The model under review builds one solid part; all positions refer to its coordinate system, in mm. A direction names the side the tool comes from. Give positions to 0.01 mm unless a question says otherwise; leave off trailing zeros. Loops run counter-clockwise (first coordinate to the right, second up) from the corner with the lowest first, then second, coordinate; pieces in that order, holes last. Notation, with made-up numbers: M 32,3 L 47,3 A31 cw 47,38 Z; hole C -5.75,78.25 d2. An arc over 180 degrees is marked long. Return JSON: item names as keys, results as strings. Group by question number.
```python
from build123d import *

# Parameters (mm, degrees)
CUT_EXTRUDE1_START     = -5
CUT_EXTRUDE1_OUTLINE_R = 1.75
CUT_EXTRUDE1_OUTLINE_W = 20.75
CUT_EXTRUDE1_OUTLINE_H = 41.25
CUT_EXTRUDE1_DEPTH     = 5
BOSS_EXTRUDE1_START    = -5
BOSS_EXTRUDE1_DEPTH    = 5
SKETCH4_W              = 30
SKETCH4_H              = 60
BOSS_EXTRUDE2_DEPTH    = 5
CUT_EXTRUDE2_REACH     = 160.193
SKETCH5_W              = 4.2
SKETCH5_H              = 20
CUT_EXTRUDE3_REACH     = 160.193
SKETCH6_R              = 1.75


with BuildPart() as part:
    # Cut-Extrude1: read off the stored shape, not the designer's step
    # Cut-Extrude1 outline → Cut-Extrude1 (new body)
    with BuildSketch(Plane(origin=(5, 0, 0), x_dir=(0, 0, -1), z_dir=(1, 0, 0)).offset(CUT_EXTRUDE1_START)):
        with BuildLine():
            Line((-6.17, -30), (6.17, -30))
            ThreePointArc((6.17, -30), (12.413752878, -27.413752878), (15, -21.17))
            Line((15, -21.17), (15, 21.17))
            ThreePointArc((15, 21.17), (12.413752878, 27.413752878), (6.17, 30))
            Line((6.17, 30), (-6.17, 30))
            ThreePointArc((-6.17, 30), (-12.413752878, 27.413752878), (-15, 21.17))
            Line((-15, 21.17), (-15, -21.17))
            ThreePointArc((-15, -21.17), (-12.413752878, -27.413752878), (-6.17, -30))
        make_face()
        with Locations((-4.875, -24.3)):
            Circle(CUT_EXTRUDE1_OUTLINE_R, mode=Mode.SUBTRACT)
        with Locations((4.875, -24.3)):
            Circle(CUT_EXTRUDE1_OUTLINE_R, mode=Mode.SUBTRACT)
        with Locations((-4.875, 24.3)):
            Circle(CUT_EXTRUDE1_OUTLINE_R, mode=Mode.SUBTRACT)
        Rectangle(CUT_EXTRUDE1_OUTLINE_W, CUT_EXTRUDE1_OUTLINE_H, mode=Mode.SUBTRACT)
        with Locations((4.875, 24.3)):
            Circle(CUT_EXTRUDE1_OUTLINE_R, mode=Mode.SUBTRACT)
    extrude(amount=CUT_EXTRUDE1_DEPTH)

    # Sketch2 → Boss-Extrude1 (add)
    with BuildSketch(Plane(origin=(5, 0, 0), x_dir=(0, 0, -1), z_dir=(1, 0, 0)).offset(BOSS_EXTRUDE1_START)):
        with BuildLine():
            Line((10.375, -20.625), (6.17, -20.625))
            Line((6.17, -20.625), (6.17, -21.93080825))
            Line((6.17, -21.93080825), (7.268440243, -21.93080825))
            Line((7.268440243, -21.93080825), (7.268440243, -27.341819789))
            Line((7.268440243, -27.341819789), (6.17, -27.341819789))
            Line((6.17, -27.341819789), (6.17, -30))
            ThreePointArc((6.17, -30), (12.413752878, -27.413752878), (15, -21.17))
            Line((15, -21.17), (15, 21.17))
            ThreePointArc((15, 21.17), (12.413752878, 27.413752878), (6.17, 30))
            Line((6.17, 30), (6.17, 26.982507006))
            Line((6.17, 26.982507006), (7.710578553, 26.982507006))
            Line((7.710578553, 26.982507006), (7.710578553, 21.584637872))
            Line((7.710578553, 21.584637872), (6.17, 21.584637872))
            Line((6.17, 21.584637872), (6.17, 20.625))
            Line((6.17, 20.625), (10.375, 20.625))
            Line((10.375, 20.625), (10.375, -20.625))
        make_face()
        with BuildLine():
            Line((-8.472684232, -21.93080825), (-6.17, -21.93080825))
            Line((-6.17, -21.93080825), (-6.17, -20.625))
            Line((-6.17, -20.625), (-10.375, -20.625))
            Line((-10.375, -20.625), (-10.375, 20.625))
            Line((-10.375, 20.625), (-6.17, 20.625))
            Line((-6.17, 20.625), (-6.17, 21.584637872))
            Line((-6.17, 21.584637872), (-7.710578553, 21.584637872))
            Line((-7.710578553, 21.584637872), (-7.710578553, 26.982507006))
            Line((-7.710578553, 26.982507006), (-6.17, 26.982507006))
            Line((-6.17, 26.982507006), (-6.17, 30))
            ThreePointArc((-6.17, 30), (-12.413752878, 27.413752878), (-15, 21.17))
            Line((-15, 21.17), (-15, -21.17))
            ThreePointArc((-15, -21.17), (-12.413752878, -27.413752878), (-6.17, -30))
            Line((-6.17, -30), (-6.17, -27.341819789))
            Line((-6.17, -27.341819789), (-8.472684232, -27.341819789))
            Line((-8.472684232, -27.341819789), (-8.472684232, -21.93080825))
        make_face()
        with BuildLine():
            Line((-15, 30), (-15, 21.17))
            ThreePointArc((-15, 21.17), (-12.413752878, 27.413752878), (-6.17, 30))
            Line((-6.17, 30), (-15, 30))
        make_face()
        with BuildLine():
            Line((15, 30), (6.17, 30))
            ThreePointArc((6.17, 30), (12.413752878, 27.413752878), (15, 21.17))
            Line((15, 21.17), (15, 30))
        make_face()
        with BuildLine():
            ThreePointArc((15, -21.17), (12.413752878, -27.413752878), (6.17, -30))
            Line((6.17, -30), (15, -30))
            Line((15, -30), (15, -21.17))
        make_face()
        with BuildLine():
            Line((-15, -30), (-6.17, -30))
            ThreePointArc((-6.17, -30), (-12.413752878, -27.413752878), (-15, -21.17))
            Line((-15, -21.17), (-15, -30))
        make_face()
    extrude(amount=BOSS_EXTRUDE1_DEPTH)

    # Sketch4 → Boss-Extrude2 (add)
    with BuildSketch(Plane.ZY):
        Polygon((-50, 50), (50, 50), (50, -50), (50, -150), (-50, -150), (-50, -50), align=None)
        Rectangle(SKETCH4_W, SKETCH4_H, mode=Mode.SUBTRACT)
    extrude(amount=-BOSS_EXTRUDE2_DEPTH)

    # Sketch5 → Cut-Extrude2 (cut, up to next)
    with BuildSketch(Plane(origin=(5, 0, 0), x_dir=(0, 0, -1), z_dir=(1, 0, 0)), mode=Mode.PRIVATE) as cut_extrude2_sk1:
        with Locations((45.1, -105)):
            Rectangle(SKETCH5_W, SKETCH5_H)
    cut_extrude2_tool1 = extrude(cut_extrude2_sk1.sketch, amount=-CUT_EXTRUDE2_REACH, mode=Mode.PRIVATE) & part.part
    # Sketch5 → Cut-Extrude2 (cut, up to next)
    with BuildSketch(Plane(origin=(5, 0, 0), x_dir=(0, 0, -1), z_dir=(1, 0, 0)), mode=Mode.PRIVATE) as cut_extrude2_sk2:
        with Locations((45.1, -50)):
            Rectangle(SKETCH5_W, SKETCH5_H)
    cut_extrude2_tool2 = extrude(cut_extrude2_sk2.sketch, amount=-CUT_EXTRUDE2_REACH, mode=Mode.PRIVATE) & part.part
    # Sketch5 → Cut-Extrude2 (cut, up to next)
    with BuildSketch(Plane(origin=(5, 0, 0), x_dir=(0, 0, -1), z_dir=(1, 0, 0)), mode=Mode.PRIVATE) as cut_extrude2_sk3:
        with Locations((45.1, 5)):
            Rectangle(SKETCH5_W, SKETCH5_H)
    cut_extrude2_tool3 = extrude(cut_extrude2_sk3.sketch, amount=-CUT_EXTRUDE2_REACH, mode=Mode.PRIVATE) & part.part
    # Sketch5 → Cut-Extrude2 (cut, up to next)
    with BuildSketch(Plane(origin=(5, 0, 0), x_dir=(0, 0, -1), z_dir=(1, 0, 0)), mode=Mode.PRIVATE) as cut_extrude2_sk4:
        with Locations((-45.1, 5)):
            Rectangle(SKETCH5_W, SKETCH5_H)
    cut_extrude2_tool4 = extrude(cut_extrude2_sk4.sketch, amount=-CUT_EXTRUDE2_REACH, mode=Mode.PRIVATE) & part.part
    # Sketch5 → Cut-Extrude2 (cut, up to next)
    with BuildSketch(Plane(origin=(5, 0, 0), x_dir=(0, 0, -1), z_dir=(1, 0, 0)), mode=Mode.PRIVATE) as cut_extrude2_sk5:
        with Locations((-45.1, -50)):
            Rectangle(SKETCH5_W, SKETCH5_H)
    cut_extrude2_tool5 = extrude(cut_extrude2_sk5.sketch, amount=-CUT_EXTRUDE2_REACH, mode=Mode.PRIVATE) & part.part
    # Sketch5 → Cut-Extrude2 (cut, up to next)
    with BuildSketch(Plane(origin=(5, 0, 0), x_dir=(0, 0, -1), z_dir=(1, 0, 0)), mode=Mode.PRIVATE) as cut_extrude2_sk6:
        with Locations((-45.1, -105)):
            Rectangle(SKETCH5_W, SKETCH5_H)
    cut_extrude2_tool6 = extrude(cut_extrude2_sk6.sketch, amount=-CUT_EXTRUDE2_REACH, mode=Mode.PRIVATE) & part.part
    add(cut_extrude2_tool1.solids().sort_by_distance((5, -105, -45.1))[0], mode=Mode.SUBTRACT)
    add(cut_extrude2_tool2.solids().sort_by_distance((5, -50, -45.1))[0], mode=Mode.SUBTRACT)
    add(cut_extrude2_tool3.solids().sort_by_distance((5, 5, -45.1))[0], mode=Mode.SUBTRACT)
    add(cut_extrude2_tool4.solids().sort_by_distance((5, 5, 45.1))[0], mode=Mode.SUBTRACT)
    add(cut_extrude2_tool5.solids().sort_by_distance((5, -50, 45.1))[0], mode=Mode.SUBTRACT)
    add(cut_extrude2_tool6.solids().sort_by_distance((5, -105, 45.1))[0], mode=Mode.SUBTRACT)

    # Sketch6 → Cut-Extrude3 (cut, up to next)
    with BuildSketch(Plane.ZY, mode=Mode.PRIVATE) as cut_extrude3_sk1:
        with Locations((45.1, -77.5)):
            Circle(SKETCH6_R)
    cut_extrude3_tool1 = extrude(cut_extrude3_sk1.sketch, amount=-CUT_EXTRUDE3_REACH, mode=Mode.PRIVATE) & part.part
    # Sketch6 → Cut-Extrude3 (cut, up to next)
    with BuildSketch(Plane.ZY, mode=Mode.PRIVATE) as cut_extrude3_sk2:
        with Locations(Location((-45.1, -77.5, 0), (0, 0, 180))):
            Circle(SKETCH6_R)
    cut_extrude3_tool2 = extrude(cut_extrude3_sk2.sketch, amount=-CUT_EXTRUDE3_REACH, mode=Mode.PRIVATE) & part.part
    # Sketch6 → Cut-Extrude3 (cut, up to next)
    with BuildSketch(Plane.ZY, mode=Mode.PRIVATE) as cut_extrude3_sk3:
        with Locations((-45.1, -22.5)):
            Circle(SKETCH6_R)
    cut_extrude3_tool3 = extrude(cut_extrude3_sk3.sketch, amount=-CUT_EXTRUDE3_REACH, mode=Mode.PRIVATE) & part.part
    # Sketch6 → Cut-Extrude3 (cut, up to next)
    with BuildSketch(Plane.ZY, mode=Mode.PRIVATE) as cut_extrude3_sk4:
        with Locations(Location((45.1, -22.5, 0), (0, 0, 180))):
            Circle(SKETCH6_R)
    cut_extrude3_tool4 = extrude(cut_extrude3_sk4.sketch, amount=-CUT_EXTRUDE3_REACH, mode=Mode.PRIVATE) & part.part
    add(cut_extrude3_tool1.solids().sort_by_distance((0, -77.5, 45.1))[0], mode=Mode.SUBTRACT)
    add(cut_extrude3_tool2.solids().sort_by_distance((0, -77.5, -45.1))[0], mode=Mode.SUBTRACT)
    add(cut_extrude3_tool3.solids().sort_by_distance((0, -22.5, -45.1))[0], mode=Mode.SUBTRACT)
    add(cut_extrude3_tool4.solids().sort_by_distance((0, -22.5, 45.1))[0], mode=Mode.SUBTRACT)


solid = part.part
```
(1) For probe 1 along Y at (x, z) = (3.95, 45.1); probe 2 along Z at (x, y) = (3.85, -77.5); probe 3 along Z at (x, y) = (0.45, 13) (3 decimals), list the stretches that pass through material, from the lowest coordinate up.
(2) Mouldability with a two-part tool opening along Z and no side actions: class faces 1 (the flat face through (2, 50, -1)), 2 (the flat face through (3, -105, -47.2)), 3 (the flat face through (2, -51, 50)) as released by +Z, released by -Z, zero draft, split by the parting line, or undercut.
(3) For pin 1 (2 mm diameter, centred on y = -77.5, z = -45.1, fed in from -X) (3 decimals), flat-tipped, find the tip position at first contact; note if it passes through.
(4) For faces 4 (the flat face through (0, -49, 1)), 5 (the flat face through (3, -105, -43)), list the 3-axis set-ups (+Z, -Z, +X, -X, +Y, -Y) from which the entire face can be reached by the end or side of a thin tool; tool diameter is ignored.
(5) Add section B-B (x = 1.8). Count the separate pieces of the cut face and the enclosed holes in it, and give its area (3 significant figures).
(6) Add section A-A (y = -105.5). Write out the cut boundary in (x, z).
Verdict:
{
 "1": {"probe 1": "y = -150 to -115, -95 to -79.25, -75.75 to -60, -40 to -24.25, -20.75 to -5, 15 to 50", "probe 2": "z = -50 to -46.85, -43.35 to 43.35, 46.85 to 50", "probe 3": "z = -50 to -47.2, -43 to -10.375, 10.375 to 43, 47.2 to 50"},
 "2": {"face 1": "zero draft", "face 2": "undercut", "face 3": "released by +Z"},
 "3": {"pin 1": "passes through"},
 "4": {"face 4": "+Z, -Z, -X, +Y, -Y", "face 5": "+X, -X"},
 "5": {"separate pieces": "1", "enclosed holes": "15", "area": "18,600 mm²"},
 "6": {"outline": "M 0,-50 L 5,-50 L 5,-47.2 L 0,-47.2 Z; M 0,-43 L 5,-43 L 5,43 L 0,43 Z; M 0,47.2 L 5,47.2 L 5,50 L 0,50 Z"}
}
